The figure shows three views and two pictorial views of one solid part (mm, origin at its lowest corner). Answer the questions. Coordinates: 2 decimals unless noted, no trailing zeros. Order: outer loops, then holes, each group sorted by start corner. A loop starts at its lowest first (then second) coordinate and runs counter-clockwise, first axis right, second up. Notation, with made-up numbers: (-11, 44.5) - (4, 44.5) arc R13 cw to (4, 52.5) - close; hole circle Ø10 at (14, 27.5). An arc over 180 degrees is marked (long way). Use one line per item in the form item = value. Start each with the question number.
Item 1: Section B-B, the plane x = 92 is taken. Write down the section's boundary in (y, z) (1 decimal), and give its area (3 significant figures).
Item 2: Each of these flat-tipped pins is pushed along its axis until it touches: pin 1 Ø5.5 at (x, z) = (24.59, 113.59) entering from -Y; pin 2 Ø3 at (x, z) = (105.59, 24.59) entering from +Y; pin 3 Ø1.5 at (x, y) = (19, 1.5) entering from -Z. Where does it stop, or does it pass through?
Item 3: Section A-A, the plane y = 1.15 is taken. Count the separate pieces of the cut face and the enclosed holes in it, and give its area (3 significant figures).
Item 4: Section C-C, the plane z = 55 is taken. Write down the section's boundary in (x, y) (1 decimal).
Item 5: Consider line 1 along X through (y, z) = (2.6, 109) (1 decimal); line 2 along Z through (x, y) = (110, 1.8) (1 decimal); line 3 along X through (y, z) = (1.4, 106.5) (1 decimal). Determine where each line is inside the solid, lowest interval first. Write a range as [from, to].
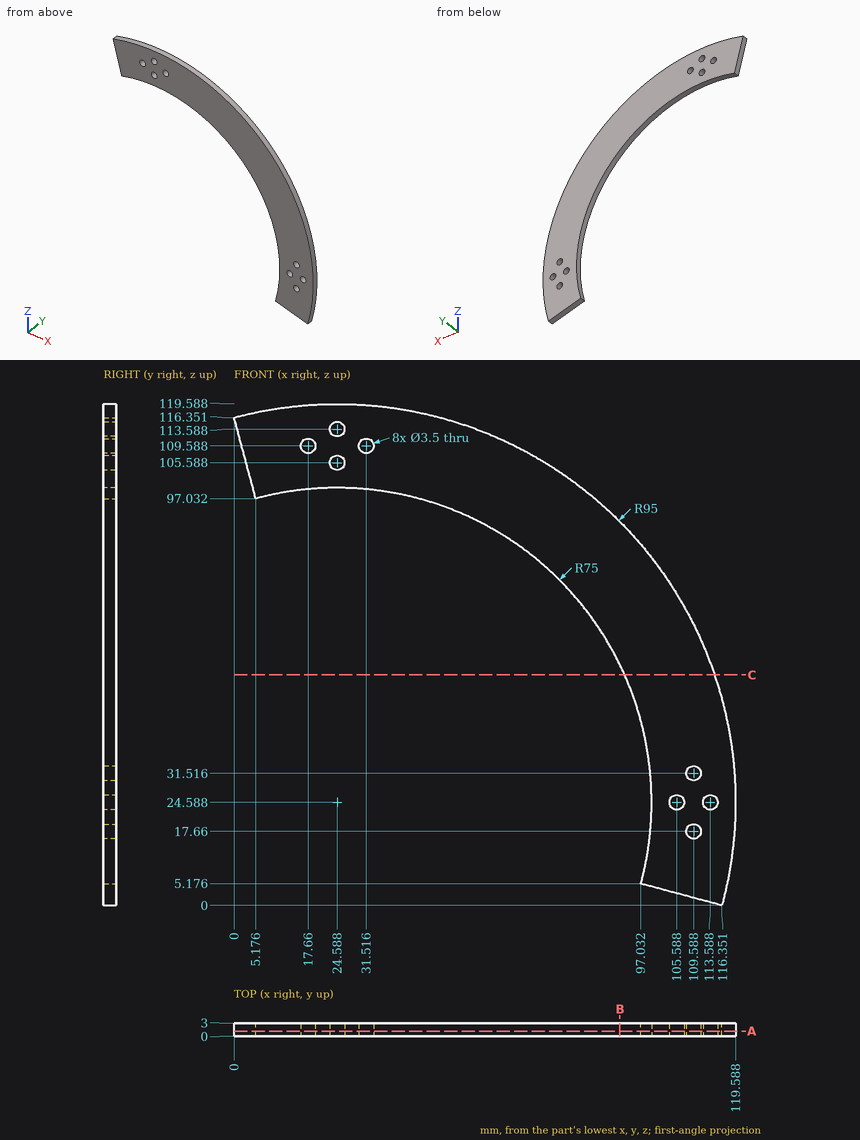
Response:
q1.outline = (0, 57.5) - (3, 57.5) - (3, 91.5) - (0, 91.5) - close
q1.area = 102 mm2
q2.pin_1 = 0
q2.pin_2 = through
q2.pin_3 = 99.32
q3.separate_pieces = 1
q3.enclosed_holes = 8
q3.area = 3,480 mm2
q4.outline = (93.1, 0) - (114.6, 0) - (114.6, 3) - (93.1, 3) - close
q5.line_1 = [2, 16], [19.3, 29.9], [33.2, 68.2]
q5.line_2 = [1.7, 16], [19.4, 29.8], [33.2, 66.2]
q5.line_3 = [2.6, 23.1], [26.1, 72.7]
